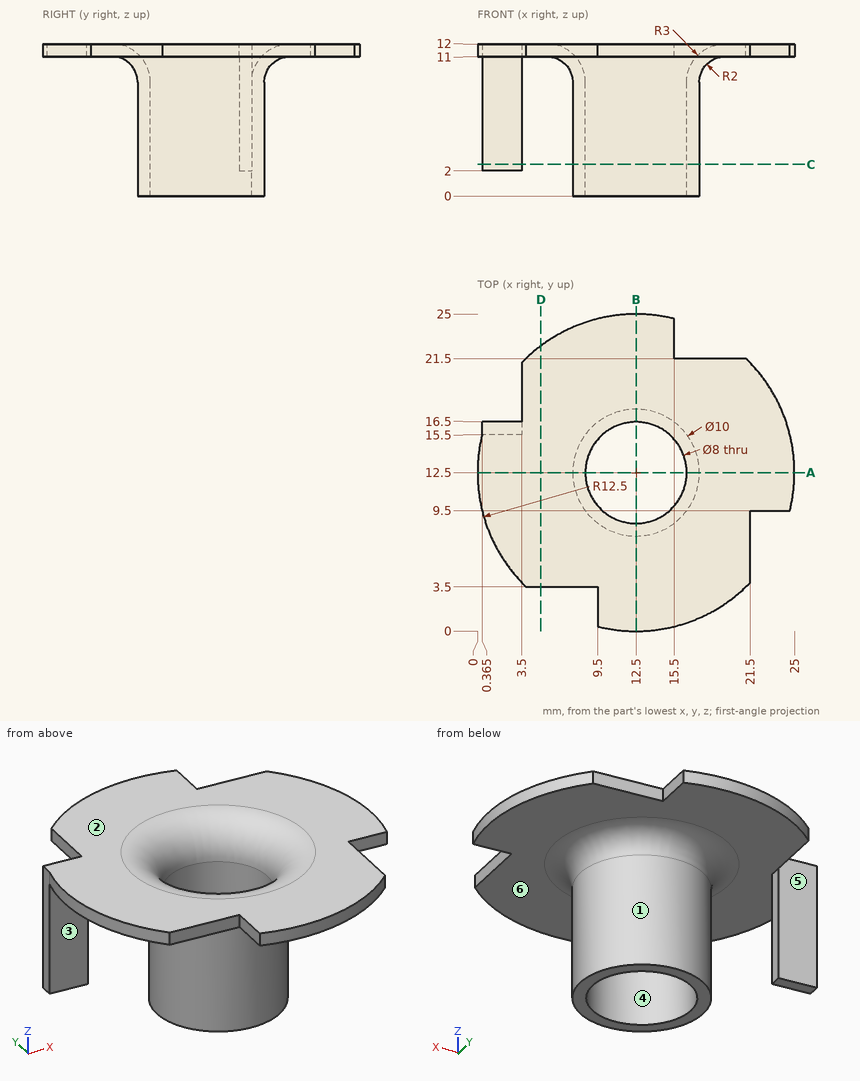
The figure shows three views and two pictorial views of one solid part (mm, origin at its lowest corner). Answer the questions. A direction names the side the tool comes from. Round coordinates to 2 decimals unless told otherwise and drop trailing zeros. Write each loop counter-clockwise with the first axis right and the second up, starting at its lowest first coordinate (ties: lowest second). Pieces come first, ordered by that corner, then holes. Notation, with made-up numbers: M 38.5,-8.5 L 91.5,-8.5 A7 ccw 91.5,-4.5 Z; hole C -13,36.5 d11. An arc over 180 degrees is marked long. Use a Markdown table: item, result.
1) A tool of negligible diameter and unlimited length cuts with its end or side. For the marked faces 1 and 2, from which of +Z, -Z, +X, -X, +Y, -Y can it reach the whole face along a straight path? Write none if from no direction.
Answers follow:
| item | result |
|---|---|
| face 1 | -Z |
| face 2 | +Z, +X, -X, +Y, -Y |
2) The part is cut by section D-D (x = 5). Write down the section's boundary in (y, z), plus the area to 3 significant figures.
Answers follow:
| item | result |
|---|---|
| outline | M 3.5,11 L 22.5,11 L 22.5,12 L 3.5,12 Z |
| area | 19.0 mm2 |
3) Flat-ended cylindrical pins translate along their axes: pin 1 (1.6 mm diameter, centred on x = 2.5, z = 7, fed in from -Y); pin 2 (4 mm diameter, centred on x = 5, z = 10, fed in from +Y); pin 3 (3.5 mm diameter, centred on x = 2, z = 6, fed in from +Y). Find the tip coordinate at first contact, or state that the pin passes through.
Answers follow:
| item | result |
|---|---|
| pin 1 | stops at y = 15.5 |
| pin 2 | stops at y = 23.59 |
| pin 3 | stops at y = 16.5 |
4) Straight lines are drawn through the part: line 1 along X through (y, z) = (12.5, 4.5); line 2 along Y through (x, z) = (9.75, 10.25). For each, find the intervals that lie inside material, in ascending order. Write a range as [from, to].
Answers follow:
| item | result |
|---|---|
| line 1 | x = [7.5, 8.5], [16.5, 17.5] |
| line 2 | y = [7.81, 9.23], [15.77, 17.19] |
5) The part is cut by section C-C (z = 2.5). Write down the section's boundary in (x, y) (1 decimal).
Answers follow:
| item | result |
|---|---|
| outline | M 0.4,15.5 L 3.5,15.5 L 3.5,16.5 L 0.4,16.5 Z; C 12.5,12.5 d10; hole C 12.5,12.5 d8 |
6) The part is cut by section A-A (y = 12.5). Write down the section's boundary in (x, z).
Answers follow:
| item | result |
|---|---|
| outline | M 0,11 L 5.5,11 A2 cw 7.5,9 L 7.5,0 L 8.5,0 L 8.5,9 A3 ccw 5.5,12 L 0,12 Z; M 16.5,0 L 17.5,0 L 17.5,9 A2 cw 19.5,11 L 25,11 L 25,12 L 19.5,12 A3 ccw 16.5,9 Z |
7) For a pull along Y with two mould halves and no side action, classify the marked faces 3, 4, 5 and 6 as pulls with the +Y half, pulls with the -Y half, needs draft (parallel to the pull), parting line crosses it, or undercut.
Answers follow:
| item | result |
|---|---|
| face 3 | pulls with the -Y half |
| face 4 | undercut |
| face 5 | pulls with the +Y half |
| face 6 | needs draft |
